from build123d import *

# Parameters (mm, degrees)
F0_W     = 79
F0_H     = 20
F1_DEPTH = 6
F2_T     = -2
F3_R     = 1
F4_R     = 0.5


with BuildPart() as f1:
    # F0 (on Front) → F1 (new body)
    with BuildSketch(Plane.XZ):
        Rectangle(F0_W, F0_H)
    extrude(amount=F1_DEPTH)

    # F2
    f2_openings = [f1.faces().sort_by_distance(p)[0] for p in [
        (0, -6, 0),
    ]]
    offset(amount=F2_T, openings=f2_openings)

    # F3
    f3_edges = [f1.edges().sort_by_distance(p)[0] for p in [
        (39.5, -3, -10),
        (-39.5, -3, -10),
        (-39.5, -3, 10),
        (39.5, -3, 10),
    ]]
    fillet(f3_edges, radius=F3_R)

    # F4
    f4_edges = [f1.edges().sort_by_distance(p)[0] for p in [
        (-37.5, -4, -8),
        (37.5, -4, -8),
        (37.5, -4, 8),
        (-37.5, -4, 8),
    ]]
    fillet(f4_edges, radius=F4_R)


solid = f1.part
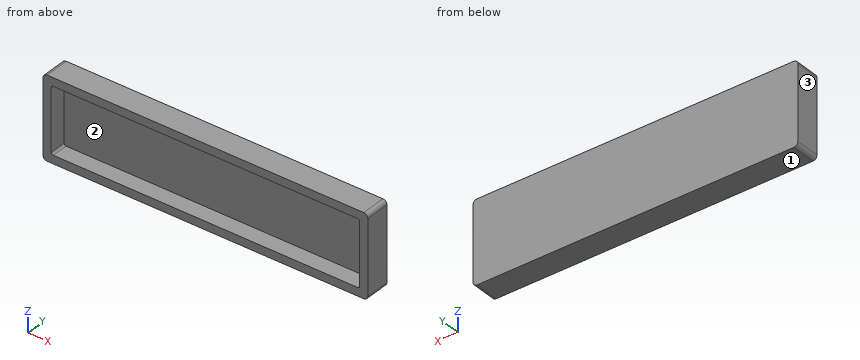
For this review, take the finished solid that the model builds, in its own axes (mm). Face numbers are marked on the shaded views. Coordinates: 2 decimals unless noted, no trailing zeros. Loops run counter-clockwise (first coordinate to the right, second up) from the corner with the lowest first, then second, coordinate; pieces in that order, holes last. Notation, with made-up numbers: (16, -31) - (42, -31) arc R19 ccw to (42, -17) - close; hole circle Ø6 at (89.5, -33.5). An arc over 180 degrees is marked (long way). Use a Markdown table: item, result. Add a question column.
Item 1: Insertion check: pin 1 Ø5 at (x, z) = (30, 5.5) entering from +Y. The pin has a flat end and moves straight along its axis. Give the tip position at first contact, or say it passes through.
Item 2: We need section C-C (x = 7). Give the boundary of the cut face in (y, z).
Item 3: For line 1 (X direction, y = -3.6, z = -5.75); line 2 (Z direction, x = -33, y = -3.85); line 3 (Y direction, x = -0.5, z = -7.25), list the stretches that pass through material, from the lowest coordinate up.
Item 4: We need section A-A (y = -3.8). Give the boundary of the cut face in (x, z), and give its area (3 significant figures).
Item 5: We need section B-B (z = 3). Give the boundary of the cut face in (x, y), and give its area (3 significant figures).
Item 6: Mouldability with a two-part tool opening along X and no side actions: class the marked faces 1, 2 and 3 as pulls with the +X half, pulls with the -X half, needs draft (parallel to the pull), parting line crosses it, or undercut.
Results list:
| question | item | result |
|---|---|---|
| 1 | pin 1 | stops at y = 0 |
| 2 | outline | (-6, -10) - (0, -10) - (0, 10) - (-6, 10) - (-6, 8) - (-2, 8) - (-2, -8) - (-6, -8) - close |
| 3 | line 1 | x = -39.5 to -37.5, 37.5 to 39.5 |
| 3 | line 2 | z = -10 to -8, 8 to 10 |
| 3 | line 3 | y = -2 to 0 |
| 4 | outline | (-39.5, -9) arc R1 ccw to (-38.5, -10) - (38.5, -10) arc R1 ccw to (39.5, -9) - (39.5, 9) arc R1 ccw to (38.5, 10) - (-38.5, 10) arc R1 ccw to (-39.5, 9) - close; hole (-37.5, -7.5) arc R0.5 ccw to (-37, -8) - (37, -8) arc R0.5 ccw to (37.5, -7.5) - (37.5, 7.5) arc R0.5 ccw to (37, 8) - (-37, 8) arc R0.5 ccw to (-37.5, 7.5) - close |
| 4 | area | 379 mm^2 |
| 5 | outline | (-39.5, -6) - (-37.5, -6) - (-37.5, -2) - (37.5, -2) - (37.5, -6) - (39.5, -6) - (39.5, 0) - (-39.5, 0) - close |
| 5 | area | 174 mm^2 |
| 6 | face 1 | needs draft |
| 6 | face 2 | undercut |
| 6 | face 3 | pulls with the -X half |
